Autodesk Fusion 360 part; units mm, degrees
sketch "Sketch1" plane through (0, 0, 0) normal (0, 1, 0) x (1, 0, 0)
  line L0 (-60, 0) -> (60, 0)
  line L1 (60, 0) -> (60, -50)
  line L2 (60, -50) -> (-60, -50)
  line L3 (-60, -50) -> (-60, 0)
  line L4 (-60, -15) -> (60, -15)
  dimension "d1" = 120
  dimension "d2" = 50
  dimension "d3" = 15
extrude "Extrude1" add sketch "Sketch1" along normal blind 15 contours L1 L2 L3 L4
extrude "Extrude2" add sketch "Sketch1" along normal blind 12 contours L0 L1 L3 L4
sketch "Sketch4" plane through (0, 0, 0) normal (0, -1, 0) x (1, 0, 0)
  line L0 (-60, 0) -> (-60, 15)
  line L1 (-60, 7.5) -> (-45, 7.5)
  line L2 (-60, 0) -> (60, 0)
  line L3 (-45, 7.5) -> (0, 7.5)
  line L4 (0, 7.5) -> (45, 7.5)
  line L5 (60, 15) -> (60, 0)
  line L6 (45, 7.5) -> (60, 7.5)
  dimension "d9" = 15
  dimension "d10" = 7.5
  dimension "d11" = 45
  dimension "d12" = 45
hole "Hole1" at (-45, 0, 7.5) at (45, 0, 7.5) at (0, 0, 7.5) direction (0, 1, 0) diameter 6.036 depth 11 tip angle 118 counterbore diameter 11 counterbore depth 7
Check sheet for the modelled part. Datum: model origin and axes. Units: mm. A direction names the side the tool comes from. Coordinates: 2 decimals unless noted, no trailing zeros. Write each loop counter-clockwise with the first axis right and the second up, starting at its lowest first coordinate (ties: lowest second). Pieces come first, ordered by that corner, then holes.
Item 1: Cross-section at B-B on y = 1.25. Record the boundary of the cut face in (x, z).
Numbers:
outline: (-60, 0) - (60, 0) - (60, 50) - (-60, 50) - close; hole circle Ø11 at (-45, 7.5); hole circle Ø11 at (0, 7.5); hole circle Ø11 at (45, 7.5)
Item 2: Depth check by flat-ended pin: pin 1 Ø4.5 at (x, z) = (14, 6.5) entering from +Y; pin 2 Ø8 at (y, z) = (12.5, 13.5) entering from -X; pin 3 Ø5.5 at (x, z) = (-47, 7.5) entering from -Y; pin 4 Ø5.5 at (x, z) = (0, 7.5) entering from -Y. Enter the tip coordinate at first touch or a pass-through.
Numbers:
pin 1: stops at y = 12
pin 2: stops at x = -60
pin 3: stops at y = 7
pin 4: stops at y = 11.16
Item 3: Cross-section at C-C on x = -45. Record the boundary of the cut face in (y, z).
Numbers:
outline: (0, 0) - (12, 0) - (12, 6.15) - (11, 4.48) - (7, 4.48) - (7, 2) - (0, 2) - close; (0, 13) - (7, 13) - (7, 10.52) - (11, 10.52) - (12, 8.85) - (12, 15) - (15, 15) - (15, 50) - (0, 50) - close
Item 4: Cross-section at A-A on z = 7.5. Count the separate pieces of the cut face and the enclosed holes in it, then the cut area to 3 significant figures.
Numbers:
separate pieces: 4
enclosed holes: 0
area: 1,120 mm2
Item 5: Mould release check, pull along X, two halves, no side actions. Record for faces 4 (the face through (-1, 6, 0)), 5 (the face through (-43, 7, 5)), 6 (the face through (-60, 7, 25)): released by +X, released by -X, zero draft, split by the parting line, or undercut.
Numbers:
face 4: zero draft
face 5: undercut
face 6: released by -X
Item 6: Scan lines: probe 1 along X at (y, z) = (4.75, 7.5); probe 2 along X at (y, z) = (8.2, 7.5); probe 3 along Z at (x, y) = (-45, 1.5). Record each from-to range of solid material in increasing order.
Numbers:
probe 1: x = -60 to -50.5, -39.5 to -5.5, 5.5 to 39.5, 50.5 to 60
probe 2: x = -60 to -48.02, -41.98 to -3.02, 3.02 to 41.98, 48.02 to 60
probe 3: z = 0 to 2, 13 to 50
Item 7: Access from +Z, -Z, +X, -X, +Y, -Y to the whole of each face (thin tool, end or side, straight path). Record for faces 1 (the face through (42.008, 9.028, 7.893)), 2 (the face through (-1, 13, 15)), 3 (the face through (-1, 15, 32)).
Numbers:
face 1: -Y
face 2: -Z, +X, -X, +Y
face 3: +Z, -Z, +X, -X, +Y
